Geometry check sheet. Reference: drawing and pictorial views, mm from the part's lowest x, y, z. A direction names the side the tool comes from. Give positions to 0.01 mm unless a question says otherwise; leave off trailing zeros. Write each loop counter-clockwise with the first axis right and the second up, starting at its lowest first coordinate (ties: lowest second). Pieces come first, ordered by that corner, then holes. Notation, with made-up numbers: M -34.5,76.25 L -22.5,76.25 A22 ccw -22.5,84.25 Z; hole C 83,87 d5. An arc over 180 degrees is marked long. Answer as a JSON object with one key per item and string values.
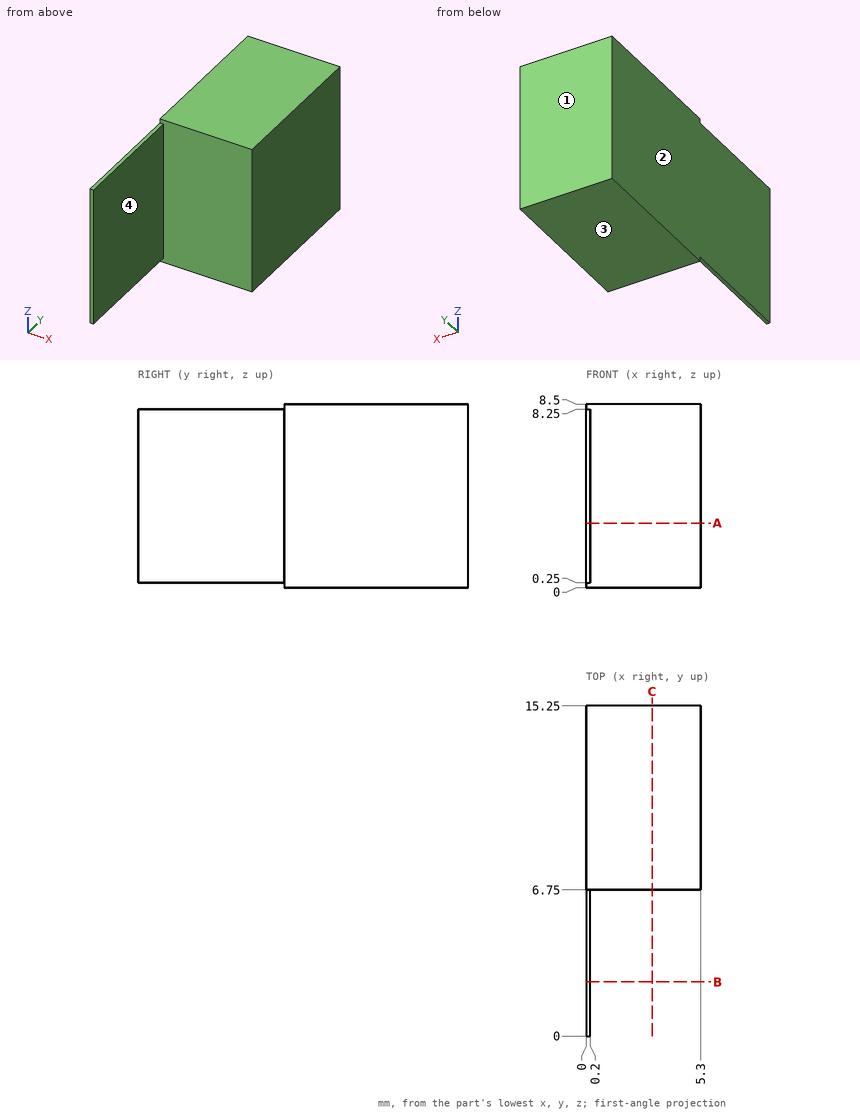
1) Go/stop test with flat-tipped pins: pin 1 (1 mm diameter, centred on x = 1, z = 3.5, fed in from -Y); pin 2 (2 mm diameter, centred on y = 3.5, z = 4, fed in from +X). Record where each tip stops, or that it passes through.
Completed:
{"pin 1": "stops at y = 6.75", "pin 2": "stops at x = 0.2"}
2) Thickness scan on L1, parallel to Y at x = 4.4, z = 7.75; L2, parallel to X at y = 1.25, z = 5. Record the ranges inside material, lowest first.
Completed:
{"L1": "y = 6.75 to 15.25", "L2": "x = 0 to 0.2"}
3) Section check B-B on y = 2.5. Record the boundary of the cut face in (x, z), and give its area (3 significant figures).
Completed:
{"outline": "M 0,0.25 L 0.2,0.25 L 0.2,8.25 L 0,8.25 Z", "area": "1.60 mm2"}
4) Section check A-A on z = 3. Record the boundary of the cut face in (x, y).
Completed:
{"outline": "M 0,0 L 0.2,0 L 0.2,6.75 L 5.3,6.75 L 5.3,15.25 L 0,15.25 Z"}
5) Access from +Z, -Z, +X, -X, +Y, -Y to the whole of each face (thin tool, end or side, straight path). Record for the marked faces 3 and 4.
Completed:
{"face 3": "-Z, +X, -X, +Y, -Y", "face 4": "+Z, -Z, +X, -Y"}
6) Release check for a two-part mould opening along Y. For the marked faces 1 and 2 record: pulls with the +Y half, pulls with the -Y half, needs draft (parallel to the pull), parting line crosses it, or undercut.
Completed:
{"face 1": "pulls with the +Y half", "face 2": "needs draft"}
7) Section check C-C on x = 3.05. Record the boundary of the cut face in (y, z).
Completed:
{"outline": "M 6.75,0 L 15.25,0 L 15.25,8.5 L 6.75,8.5 Z"}
